Check sheet for the drawn part. Datum: minimum x, y, z corner. Units: mm. A direction names the side the tool comes from. Round coordinates to 2 decimals unless told otherwise and drop trailing zeros. Write each loop counter-clockwise with the first axis right and the second up, starting at its lowest first coordinate (ties: lowest second). Pieces come first, ordered by that corner, then holes. Notation, with made-up numbers: (19, 60) - (44, 60) arc R9 cw to (44, 70) - close; hole circle Ø6 at (7.25, 65). An arc over 180 degrees is marked (long way). Answer as a JSON object with one key per item and string values. Group by question number.
Item 1: Sectioned sample at C-C on x = 27. Record the boundary of the cut face in (y, z) (1 decimal).
Item 2: Sectioned sample at A-A on z = 10.25. Record the boundary of the cut face in (x, y) (1 decimal).
Item 3: Thickness scan on line 1 (X direction, y = 1.05, z = 8.5) (1 decimal); line 2 (Z direction, x = 3.5, y = 2.1). Record the ranges inside material, lowest first.
Item 4: Set-up check for the marked faces 1, 2 and 3: record each of +Z, -Z, +X, -X, +Y, -Y from which the full face is reachable in a straight line by a thin tool's end or side.
Item 5: Gauge pin test, flat ends, axial feed: P1, Ø1, axis at x = 24.5, y = 2, coming from the -Z side; P2, Ø1.3, axis at y = 1.5, z = 0.5, coming from the +X side (1 decimal); P3, Ø1.6, axis at x = 3.5, y = 2, coming from the +Z side. Record the tip position at first contact, or that the pin passes through.
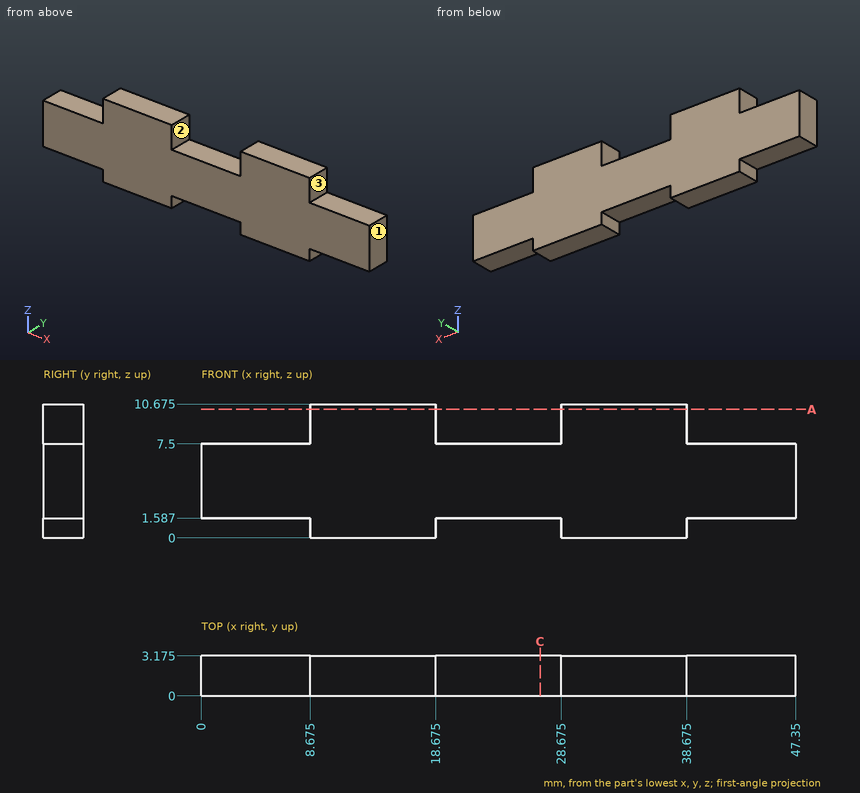
Completed:
{
 "1": {"outline": "(0, 1.6) - (3.2, 1.6) - (3.2, 7.5) - (0, 7.5) - close"},
 "2": {"outline": "(8.7, 0) - (18.7, 0) - (18.7, 3.2) - (8.7, 3.2) - close; (28.7, 0) - (38.7, 0) - (38.7, 3.2) - (28.7, 3.2) - close"},
 "3": {"line 1": "8.7 to 18.7, 28.7 to 38.7", "line 2": "1.59 to 7.5"},
 "4": {"face 1": "+Z, -Z, +X, +Y, -Y", "face 2": "+Z, +Y, -Y", "face 3": "+Z, +X, +Y, -Y"},
 "5": {"P1": "z = 1.59", "P2": "x = 38.7", "P3": "z = 7.5"}
}
